Input: part model. Units: mm. Frame: model coordinates. A direction names the side the tool comes from. Coordinates: 2 decimals unless noted, no trailing zeros. Order: outer loops, then holes, each group sorted by start corner. A loop starts at its lowest first (then second) coordinate and runs counter-clockwise, first axis right, second up. Notation, with made-up numbers: M 36,-1.5 L 76,-1.5 A26 cw 76,21.5 Z; hole C -9.5,-35 d8. An arc over 180 degrees is marked long. One line per item, written item: value.
```python
from build123d import *

# Parameters (mm, degrees)
BOSS_EXTRUDE1_DEPTH = 1.5
SKETCH2_R           = 2.5
BOSS_EXTRUDE2_DEPTH = 1.5
SKETCH3_R           = 2.35
CUT_EXTRUDE1_DEPTH  = 2
SKETCH4_R           = 0.5
CUT_EXTRUDE2_DEPTH  = 2


with BuildPart() as part:
    # Sketch1 → Boss-Extrude1 (new body)
    with BuildSketch(Plane.XY):
        with BuildLine():
            Line((-1.5, 16), (-2.495083503, 0.156710922))
            ThreePointArc((-2.495083503, 0.156710922), (0, -2.5), (2.495083503, 0.156710922))
            Line((2.495083503, 0.156710922), (1.5, 16))
            ThreePointArc((1.5, 16), (0, 17.5), (-1.5, 16))
        make_face()
    extrude(amount=BOSS_EXTRUDE1_DEPTH)

    # Sketch2 → Boss-Extrude2 (add)
    with BuildSketch(Plane.XY.offset(1.5)):
        Circle(SKETCH2_R)
    extrude(amount=BOSS_EXTRUDE2_DEPTH)

    # Sketch3 → Cut-Extrude1 (cut)
    with BuildSketch(Plane.XY.offset(3)):
        Circle(SKETCH3_R)
    extrude(amount=-CUT_EXTRUDE1_DEPTH, mode=Mode.SUBTRACT)

    # Sketch4 → Cut-Extrude2 (cut)
    with BuildSketch(Plane.XY.offset(1.5)):
        with Locations((0, 16)):
            Circle(SKETCH4_R)
    extrude(amount=-CUT_EXTRUDE2_DEPTH, mode=Mode.SUBTRACT)


solid = part.part
```
(1) Cut plane C-C on y = 16.25. Output: boundary loops of the cut face in (x, z).
Data:
outline: M -1.48,0 L -0.43,0 L -0.43,1.5 L -1.48,1.5 Z; M 0.43,0 L 1.48,0 L 1.48,1.5 L 0.43,1.5 Z
(2) Access query for faces 1 (the flat face through (0, 0, 1)), 2 (the flat face through (2.005, 7.967, 0.74)). Directions: +Z, -Z, +X, -X, +Y, -Y. A direction counts if a zero-diameter tool reaches every point of the face in a straight line with its end or side. Return the directions, or none.
Data:
face 1: +Z
face 2: +Z, -Z, +X, +Y
(3) Cut plane D-D on x = 1.3. Output: boundary loops of the cut face in (y, z), plus the area to 3 significant figures.
Data:
outline: M -2.14,0 L 16.75,0 L 16.75,1.5 L 2.14,1.5 L 2.14,3 L 1.96,3 L 1.96,1 L -1.96,1 L -1.96,3 L -2.14,3 Z
area: 26.9 mm2
(4) First-contact query: pin 1 (1 mm diameter, centred on y = 9, z = 1, fed in from +X); pin 2 (2.5 mm diameter, centred on x = 0, y = -0.5, fed in from +Z); pin 3 (2.5 mm diameter, centred on x = 0, y = 6.5, fed in from +Z). Flat tips, straight axial feed; report the tip coordinate or a pass-through.
Data:
pin 1: stops at x = 1.97
pin 2: stops at z = 1
pin 3: stops at z = 1.5
(5) Draft query along Y for faces 3 (the flat face through (0, 8, 0)), 4 (the cylindrical face through (-0.509, -2.294, 2.014)), 5 (the flat face through (-1.99, 8.19, 0.74)). Return one class per face: released by +Y, released by -Y, zero draft, split by the parting line, or undercut.
Data:
face 3: zero draft
face 4: undercut
face 5: released by +Y
(6) Ray query, line 1 (Y direction, x = 0, z = 1.05); line 2 (Y direction, x = -0.15, z = 1.6); line 3 (Y direction, x = 0, z = 0.9). Return the intervals inside material, ascending. Write a range as from..to.
Data:
line 1: y = -2.5..-2.35, 2.35..15.5, 16.5..17.5
line 2: y = -2.5..-2.35, 2.35..2.5
line 3: y = -2.5..15.5, 16.5..17.5
(7) Cut plane A-A on x = 0. Output: boundary loops of the cut face in (y, z).
Data:
outline: M -2.5,0 L 15.5,0 L 15.5,1.5 L 2.5,1.5 L 2.5,3 L 2.35,3 L 2.35,1 L -2.35,1 L -2.35,3 L -2.5,3 Z; M 16.5,0 L 17.5,0 L 17.5,1.5 L 16.5,1.5 Z
